```python
from build123d import *

# Parameters (mm, degrees)
F0_W     = 72.709278
F0_H     = 139.160782
F1_DEPTH = 38.1
F2_W     = 63.17363
F2_H     = 130.221114
F3_DEPTH = 76.201
F4_R     = 12.32698
F5_DEPTH = 139.161782
F6_W     = 29.30933
F6_H     = 123.367376
F7_DEPTH = 72.710277


with BuildPart() as f1:
    # F0 (on Front) → F1 (new body, symmetric)
    with BuildSketch(Plane.XZ):
        Rectangle(F0_W, F0_H)
    extrude(amount=F1_DEPTH, both=True)

    # F2 (on face) → F3 (cut, through all)
    with BuildSketch(Plane.XZ.offset(38.1)):
        Rectangle(F2_W, F2_H)
    extrude(amount=-F3_DEPTH, mode=Mode.SUBTRACT)

    # F4 (on face) → F5 (cut, through all)
    with BuildSketch(Plane.XY.offset(69.580391)):
        Circle(F4_R)
    extrude(amount=-F5_DEPTH, mode=Mode.SUBTRACT)

    # F6 (on face) → F7 (cut, through all)
    with BuildSketch(Plane(origin=(-36.354639, 0, 0), x_dir=(0, -1, 0), z_dir=(-1, 0, 0))):
        with Locations((-23.445335, 0)):
            Rectangle(F6_W, F6_H)
        with Locations((-52.754665, 0)):
            Rectangle(F6_W, F6_H)
    extrude(amount=-F7_DEPTH, mode=Mode.SUBTRACT)


solid = f1.part
```
Input: part model. Units: mm. Frame: model coordinates. A direction names the side the tool comes from. Round coordinates to 2 decimals unless told otherwise and drop trailing zeros. Order: outer loops, then holes, each group sorted by start corner. A loop starts at its lowest first (then second) coordinate and runs counter-clockwise, first axis right, second up. Notation, with made-up numbers: (-26, 35) - (32, 35) arc R32 cw to (32, 65) - close; hole circle Ø4 at (57.5, 89). An arc over 180 degrees is marked (long way). Answer in a Markdown table with one row per item.
Item 1: Line query: line 1 (Z direction, x = -29.5, y = 26.5); line 2 (Y direction, x = 0, z = -68); line 3 (X direction, y = -14, z = -51.5). Output: solid intervals per line, ascending.
Model answer:
| item | result |
|---|---|
| line 1 | z = -69.58 to -65.11, 65.11 to 69.58 |
| line 2 | y = -38.1 to -12.33, 12.33 to 38.1 |
| line 3 | x = -36.35 to -31.59, 31.59 to 36.35 |
Item 2: Section query C-C (x = 0). Return the cut outline in (y, z), then the cut area to 3 significant figures.
Model answer:
| item | result |
|---|---|
| outline | (-38.1, -69.58) - (-12.33, -69.58) - (-12.33, -65.11) - (-38.1, -65.11) - close; (-38.1, 65.11) - (-12.33, 65.11) - (-12.33, 69.58) - (-38.1, 69.58) - close; (12.33, -69.58) - (38.1, -69.58) - (38.1, -65.11) - (12.33, -65.11) - close; (12.33, 65.11) - (38.1, 65.11) - (38.1, 69.58) - (12.33, 69.58) - close |
| area | 461 mm² |
Item 3: Pin query (flat end, axial travel): pin 1 (1.4 mm diameter, centred on x = -33, z = -10, fed in from +Y). Return the tip coordinate at first contact, or that it passes through.
Model answer:
| item | result |
|---|---|
| pin 1 | stops at y = 8.79 |
Item 4: Section query D-D (y = 0). Return the cut outline in (x, z).
Model answer:
| item | result |
|---|---|
| outline | (-36.35, -69.58) - (-12.33, -69.58) - (-12.33, -65.11) - (-31.59, -65.11) - (-31.59, 65.11) - (-12.33, 65.11) - (-12.33, 69.58) - (-36.35, 69.58) - close; (12.33, -69.58) - (36.35, -69.58) - (36.35, 69.58) - (12.33, 69.58) - (12.33, 65.11) - (31.59, 65.11) - (31.59, -65.11) - (12.33, -65.11) - close |
Item 5: Section query A-A (y = -25.5). Return the cut outline in (x, z).
Model answer:
| item | result |
|---|---|
| outline | (-36.35, -69.58) - (36.35, -69.58) - (36.35, 69.58) - (-36.35, 69.58) - close; hole (-31.59, -65.11) - (31.59, -65.11) - (31.59, 65.11) - (-31.59, 65.11) - close |
Item 6: Reachability of faces 5 (the flat face through (-1, 38.1, 67)), 6 (the flat face through (-31.587, -17, -1)), 7 (the flat face through (-34, 8.791, -1)) from +Z, -Z, +X, -X, +Y, -Y: full face, straight path, thin tool, end or side. Return the list, or none.
Model answer:
| item | result |
|---|---|
| face 5 | +Z, -Z, +X, -X, +Y |
| face 6 | +Y, -Y |
| face 7 | +X, -X, +Y |
Item 7: Section query B-B (z = -33). Return the cut outline in (x, y), then the cut area to 3 significant figures.
Model answer:
| item | result |
|---|---|
| outline | (-36.35, -38.1) - (-31.59, -38.1) - (-31.59, 8.79) - (-36.35, 8.79) - close; (31.59, -38.1) - (36.35, -38.1) - (36.35, 8.79) - (31.59, 8.79) - close |
| area | 447 mm² |
Item 8: Mould query, pull axis X, two halves, no side actions, for faces 1 (the flat face through (14, -1, 65.111)), 2 (the flat face through (-34, 23, 61.684)), 3 (the flat face through (36.355, -9, -1)), 4 (the flat face through (-36.355, -9, -1)). Classes: released by +X, released by -X, zero draft, split by the parting line, or undercut.
Model answer:
| item | result |
|---|---|
| face 1 | undercut |
| face 2 | zero draft |
| face 3 | released by +X |
| face 4 | released by -X |
